from build123d import *

# Parameters (mm, degrees)
SKETCH1_W                 = 387.38683
SKETCH1_H                 = 391.2598474
BOSS_EXTRUDE1_DEPTH       = 0.035
FILLET1_R                 = 11.811
CONVERT_SOLID1_START      = -0.854
CONVERT_SOLID1_DEPTH      = 0.854
EDGE_FLANGE1_DEPTH        = 367.6378474
EDGE_FLANGE1_BEND_DEPTH   = 363.76483
EDGE_FLANGE1_BEND_2_DEPTH = 367.6378474
EDGE_FLANGE1_BEND_3_DEPTH = 363.76483


# Read off the part's stored shape, not the designer's step: Convert-Solid1
# Sheet-metal steps are written as plain solids
with BuildPart() as part:
    # Sketch1 → Boss-Extrude1 (new body)
    with BuildSketch(Plane(origin=(0, 0, 0), x_dir=(1, 0, 0), z_dir=(0, 1, 0))):
        Rectangle(SKETCH1_W, SKETCH1_H)
    extrude(amount=BOSS_EXTRUDE1_DEPTH)

    # Fillet1
    fillet1_edges = [part.edges().sort_by_distance(p)[0] for p in [
        (193.693415, 0.0175, -195.6299237),
        (193.693415, 0.0175, 195.6299237),
        (-193.693415, 0.0175, 195.6299237),
        (-193.693415, 0.0175, -195.6299237),
    ]]
    fillet(fillet1_edges, radius=FILLET1_R)

    # Convert-Solid1 outline → Convert-Solid1 (add)
    with BuildSketch(Plane(origin=(0, 0, 0), x_dir=(1, 0, 0), z_dir=(0, 1, 0)).offset(CONVERT_SOLID1_START)):
        with BuildLine():
            ThreePointArc((193.693415, 183.8189237), (190.234053193, 192.170561893), (181.882415, 195.6299237))
            Line((181.882415, 195.6299237), (-181.882415, 195.6299237))
            ThreePointArc((-181.882415, 195.6299237), (-190.234053193, 192.170561893), (-193.693415, 183.8189237))
            Line((-193.693415, 183.8189237), (-193.693415, -183.8189237))
            ThreePointArc((-193.693415, -183.8189237), (-190.234053193, -192.170561893), (-181.882415, -195.6299237))
            Line((-181.882415, -195.6299237), (181.882415, -195.6299237))
            ThreePointArc((181.882415, -195.6299237), (190.234053193, -192.170561893), (193.693415, -183.8189237))
            Line((193.693415, -183.8189237), (193.693415, 183.8189237))
        make_face()
    extrude(amount=CONVERT_SOLID1_DEPTH)

    # Edge-Flange1 section (across the edge) → Edge-Flange1 (add)
    with BuildSketch(Plane(origin=(-194.074415, -0.854, 183.8189237), x_dir=(1, 0, 0), z_dir=(0, 0, -1))):
        with BuildLine():
            Line((-0.889, 0.381), (-0.889, 15))
            Line((-0.889, 15), (0, 15))
            Line((0, 15), (0, 0.381))
            ThreePointArc((0, 0.381), (0.111592316, 0.111592316), (0.381, 0))
            Line((0.381, 0), (0.381, -0.889))
            ThreePointArc((0.381, -0.889), (-0.517025612, -0.517025612), (-0.889, 0.381))
        make_face()
    extrude(amount=EDGE_FLANGE1_DEPTH)

    # Edge-Flange1 section 2 (across the edge) → Edge-Flange1 bend (add)
    with BuildSketch(Plane(origin=(181.882415, -0.854, 196.0109237), x_dir=(0, 0, -1), z_dir=(-1, 0, 0))):
        with BuildLine():
            Line((-0.889, 0.381), (-0.889, 15))
            Line((-0.889, 15), (0, 15))
            Line((0, 15), (0, 0.381))
            ThreePointArc((0, 0.381), (0.111592316, 0.111592316), (0.381, 0))
            Line((0.381, 0), (0.381, -0.889))
            ThreePointArc((0.381, -0.889), (-0.517025612, -0.517025612), (-0.889, 0.381))
        make_face()
    extrude(amount=EDGE_FLANGE1_BEND_DEPTH)

    # Edge-Flange1 section 3 (across the edge) → Edge-Flange1 bend 2 (add)
    with BuildSketch(Plane(origin=(194.074415, -0.854, -183.8189237), x_dir=(-1, 0, 0), z_dir=(0, 0, 1))):
        with BuildLine():
            Line((-0.889, 0.381), (-0.889, 15))
            Line((-0.889, 15), (0, 15))
            Line((0, 15), (0, 0.381))
            ThreePointArc((0, 0.381), (0.111592316, 0.111592316), (0.381, 0))
            Line((0.381, 0), (0.381, -0.889))
            ThreePointArc((0.381, -0.889), (-0.517025612, -0.517025612), (-0.889, 0.381))
        make_face()
    extrude(amount=EDGE_FLANGE1_BEND_2_DEPTH)

    # Edge-Flange1 section 4 (across the edge) → Edge-Flange1 bend 3 (add)
    with BuildSketch(Plane(origin=(-181.882415, -0.854, -196.0109237), x_dir=(0, 0, 1), z_dir=(1, 0, 0))):
        with BuildLine():
            Line((-0.889, 0.381), (-0.889, 15))
            Line((-0.889, 15), (0, 15))
            Line((0, 15), (0, 0.381))
            ThreePointArc((0, 0.381), (0.111592316, 0.111592316), (0.381, 0))
            Line((0.381, 0), (0.381, -0.889))
            ThreePointArc((0.381, -0.889), (-0.517025612, -0.517025612), (-0.889, 0.381))
        make_face()
    extrude(amount=EDGE_FLANGE1_BEND_3_DEPTH)


solid = part.part
The listing builds one solid part. Answer for the finished solid, in the listing's coordinates (mm). A direction names the side the tool comes from. Round coordinates to 2 decimals unless told otherwise and drop trailing zeros. Order: outer loops, then holes, each group sorted by start corner. A loop starts at its lowest first (then second) coordinate and runs counter-clockwise, first axis right, second up. Notation, with made-up numbers: (-23, -2) -> (28, -2) arc R13 ccw to (28, 22) -> close; hole circle Ø7 at (35.25, -4). An arc over 180 degrees is marked (long way). Put each result on its own line as item: value.
Q1. Which of the six approach directions +Z, -Z, +X, -X, +Y, -Y give full straight-line access (tool end or side, diameter ignored) to faces 1 (the flat face through (194.074, -9, -3)), 2 (the flat face through (-3, -8, -196.9)), 3 (the flat face through (-3, -9, -196.011)), 4 (the flat face through (-3, -0.854, -3))?
Results list:
face 1: +Z, -Z, -Y
face 2: -Z, +X, -X, +Y, -Y
face 3: +X, -X, -Y
face 4: -Y
Q2. Determine the mould class of faces 5 (the flat face through (3, -8, 196.9)), 6 (the flat face through (-3, 0.035, -3)), 7 (the flat face through (3, -9, 196.011)) for opening direction Z: pulls with the +Z half, pulls with the -Z half, needs draft (parallel to the pull), parting line crosses it, or undercut.
Results list:
face 5: pulls with the +Z half
face 6: needs draft
face 7: undercut
Q3. Each of these flat-tipped pins is pushed along its axis until it touches: P1, Ø1.4, axis at x = 194, y = -9, coming from the +Z side; P2, Ø1.4, axis at y = -5.5, z = 196, coming from the -X side; P3, Ø1, axis at y = -4.5, z = 196, coming from the +X side. Where does it stop, or does it pass through?
Results list:
P1: z = 183.82
P2: x = -181.88
P3: x = 181.88
Q4. Consider line 1 along Z through (x, y) = (-147.5, -7.5); line 2 along X through (y, z) = (-14, 115.5); line 3 along X through (y, z) = (-1, 16). Determine where each line is inside the solid, lowest interval first.
Results list:
line 1: -196.9 to -196.01, 196.01 to 196.9
line 2: -194.96 to -194.07, 194.07 to 194.96
line 3: -194.94 to -193.99, 193.99 to 194.94
Q5. Section C-C, the plane z = -168 is taken. Write down the section's boundary in (x, y) (3 decimals).
Results list:
outline: (-194.963, -15.854) -> (-194.074, -15.854) -> (-194.074, -1.235) arc R0.381 cw to (-193.693, -0.854) -> (193.693, -0.854) arc R0.381 cw to (194.074, -1.235) -> (194.074, -15.854) -> (194.963, -15.854) -> (194.963, -1.235) arc R1.27 ccw to (193.693, 0.035) -> (-193.693, 0.035) arc R1.27 ccw to (-194.963, -1.235) -> close
Q6. Section B-B, the plane x = 11 is taken. Write down the section's boundary in (y, z) (3 decimals).
Results list:
outline: (-15.854, -196.9) -> (-1.235, -196.9) arc R1.27 ccw to (0.035, -195.63) -> (0.035, 195.63) arc R1.27 ccw to (-1.235, 196.9) -> (-15.854, 196.9) -> (-15.854, 196.011) -> (-1.235, 196.011) arc R0.381 cw to (-0.854, 195.63) -> (-0.854, -195.63) arc R0.381 cw to (-1.235, -196.011) -> (-15.854, -196.011) -> close
Q7. Section A-A, the plane y = -7.25 is taken. Write down the section's boundary in (x, z), and give its area (3 significant figures).
Results list:
outline: (-194.96, -183.82) -> (-194.07, -183.82) -> (-194.07, 183.82) -> (-194.96, 183.82) -> close; (-181.88, -196.9) -> (181.88, -196.9) -> (181.88, -196.01) -> (-181.88, -196.01) -> close; (-181.88, 196.01) -> (181.88, 196.01) -> (181.88, 196.9) -> (-181.88, 196.9) -> close; (194.07, -183.82) -> (194.96, -183.82) -> (194.96, 183.82) -> (194.07, 183.82) -> close
area: 1,300 mm^2
